Could you check a few things on this model? Use its own coordinates, in mm. Face numbers are marked on the shaded views. A direction names the side the tool comes from. Give positions to 0.01 mm unless a question says otherwise; leave off trailing zeros. Write each loop counter-clockwise with the first axis right and the second up, starting at its lowest first coordinate (ties: lowest second). Pieces come first, ordered by that corner, then holes. Notation, with made-up numbers: M 16,13 L 37,13 A31 ccw 37,39 Z; hole C 52,85 d7. An arc over 180 degrees is marked long. Use one line per item in the form item = value.
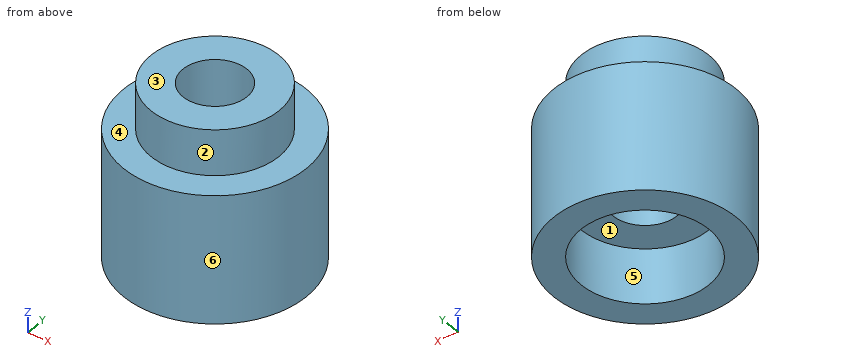
Autodesk Fusion 360 part; units mm, degrees
sketch "Skizze1" plane through (0, 0, 0) normal (0, 0, 1) x (1, 0, 0)
  line L0 (-31.5508, 0) -> (33.8224, 0) construction
  line L1 (0, 25.6192) -> (0, -38.4919) construction
  circle A0 centre (0, 0) radius 1.75
  circle A1 centre (0, 0) radius 3.5
  circle A2 centre (0, 0) radius 5
  dimension "d1" = 3.5
  dimension "d2" = 7
  dimension "d3" = 10
extrude "Extrusion1" add sketch "Skizze1" along normal blind 7 contours A1 | A2
extrude "Extrusion2" add sketch "Skizze1" along normal blind 9.5 contours A1
extrude "Extrusion3" cut sketch "Skizze1" along normal blind 3 contours A1
1) I want a section at A-A, the plane y = 0. Please give me the cut outline in (x, z), plus the area to 4 significant figures.
Checked values:
outline = M -5,0 L -3.5,0 L -3.5,3 L -1.75,3 L -1.75,9.5 L -3.5,9.5 L -3.5,7 L -5,7 Z; M 1.75,3 L 3.5,3 L 3.5,0 L 5,0 L 5,7 L 3.5,7 L 3.5,9.5 L 1.75,9.5 Z
area = 43.75 mm2
2) For the marked faces 4, 5 and 6, which set-ups out of +Z, -Z, +X, -X, +Y, -Y let a thin tool reach every point of the face, with its end or its side?
Checked values:
face_4 = +Z
face_5 = -Z
face_6 = +Z, -Z
3) I want a section at C-C, the plane z = 4. Please give me the cut outline in (x, y), plus the area to 3 significant figures.
Checked values:
outline = C 0,0 d10; hole C 0,0 d3.5
area = 68.9 mm2
4) I want a section at D-D, the plane x = -2.5. Please give me the cut outline in (y, z).
Checked values:
outline = M -4.33,0 L -2.45,0 L -2.45,3 L 2.45,3 L 2.45,0 L 4.33,0 L 4.33,7 L 2.45,7 L 2.45,9.5 L -2.45,9.5 L -2.45,7 L -4.33,7 Z
5) Thinking about a two-plate mould opening in Y: for the marked faces 1, 2 and 3, which applies, released by +Y, released by -Y, zero draft, split by the parting line, or undercut?
Checked values:
face_1 = undercut
face_2 = split by the parting line
face_3 = zero draft
6) For pin 1 Ø2 at (x, y) = (0, 0) entering from +Z, with a flat end and sliding along its axis, tell me the tip position at first contact or that it passes through.
Checked values:
pin_1 = through
7) If I drill on L1, parallel to Y at x = 0, z = 7.25; L2, parallel to Y at x = 0, z = 5.75; L3, parallel to Z at x = -2, y = -4.5, over which ranges is the centre line in solid material (lowest first)?
Checked values:
L1 = -3.5 to -1.75, 1.75 to 3.5
L2 = -5 to -1.75, 1.75 to 5
L3 = 0 to 7
